Input: part model. Units: mm. Frame: model coordinates. A direction names the side the tool comes from. Coordinates: 2 decimals unless noted, no trailing zeros. Write each loop counter-clockwise with the first axis right and the second up, starting at its lowest first coordinate (ties: lowest second). Pieces come first, ordered by that corner, then holes.
1) Section query A-A (x = 0). Output: boundary loops of the cut face in (y, z).
2) Pin query (flat end, axial travel): pin 1 Ø1.8 at (x, y) = (5.66, -5.66) entering from -Z; pin 2 Ø2 at (x, y) = (7.5, -4.5) entering from +Z. Return the tip coordinate at first contact, or that it passes through.
3) Section query D-D (y = -6.75). State how many separate pieces and enclosed holes the cut face has, then the cut area to 3 significant figures.
4) Set-up query: faces 4 (the flat face through (0, -7, 2)), 5 (the flat face through (0, 3, 0)). Return all of +Z, -Z, +X, -X, +Y, -Y with unobstructed straight access to the full face (end or side cutting, diameter ignored); none if empty.
5) Line query: L1, parallel to Y at x = 0, z = 3; L2, parallel to Z at x = -3.5, y = 6.75; L3, parallel to Y at x = 0.5, z = 3. Output: solid intervals per line, ascending.
6) Section query C-C (z = 4.5). Output: boundary loops of the cut face in (x, y), then the cut area to 3 significant figures.
7) Draft query along X for faces 1 (the flat face through (1, -3, 12)), 2 (the cylindrical face through (-2.38, -10.74, 0.74)), 3 (the cylindrical face through (-4.225, 6.108, 0.986)). Return one class per face: pulls with the +X half, pulls with the -X half, needs draft (parallel to the pull), parting line crosses it, or undercut.
from build123d import *

# Parameters (mm, degrees)
SKETCH1_R           = 11
SKETCH1_R_2         = 2.5
SKETCH1_R_3         = 1.5
BOSS_EXTRUDE1_DEPTH = 2
SKETCH2_R           = 5
SKETCH2_R_2         = 2.5
BOSS_EXTRUDE2_DEPTH = 10
FILLET1_R           = 0.5


with BuildPart() as part:
    # Sketch1 → Boss-Extrude1 (new body)
    with BuildSketch(Plane.XY):
        Circle(SKETCH1_R)
        Circle(SKETCH1_R_2, mode=Mode.SUBTRACT)
        with Locations((-5.655999742, 5.657708628)):
            Circle(SKETCH1_R_3, mode=Mode.SUBTRACT)
        with Locations((5.655999742, 5.657708628)):
            Circle(SKETCH1_R_3, mode=Mode.SUBTRACT)
        with Locations((5.655999742, -5.657708628)):
            Circle(SKETCH1_R_3, mode=Mode.SUBTRACT)
        with Locations((-5.655999742, -5.657708628)):
            Circle(SKETCH1_R_3, mode=Mode.SUBTRACT)
    extrude(amount=BOSS_EXTRUDE1_DEPTH)

    # Sketch2 → Boss-Extrude2 (add)
    with BuildSketch(Plane.XY.offset(2)):
        Circle(SKETCH2_R)
        Circle(SKETCH2_R_2, mode=Mode.SUBTRACT)
    extrude(amount=BOSS_EXTRUDE2_DEPTH)

    # Fillet1
    fillet1_edges = [part.edges().sort_by_distance(p)[0] for p in [
        (-5, 0, 12),
        (-5, 0, 2),
        (-2.5, 0, 12),
        (-11, 0, 2),
    ]]
    fillet(fillet1_edges, radius=FILLET1_R)


solid = part.part
Answer:
1. outline: (-11, 0) - (-2.5, 0) - (-2.5, 11.5) arc R0.5 ccw to (-3, 12) - (-4.5, 12) arc R0.5 ccw to (-5, 11.5) - (-5, 2.5) arc R0.5 cw to (-5.5, 2) - (-10.5, 2) arc R0.5 ccw to (-11, 1.5) - close; (2.5, 0) - (11, 0) - (11, 1.5) arc R0.5 ccw to (10.5, 2) - (5.5, 2) arc R0.5 cw to (5, 2.5) - (5, 11.5) arc R0.5 ccw to (4.5, 12) - (3, 12) arc R0.5 ccw to (2.5, 11.5) - close
2. pin 1: passes through
2. pin 2: stops at z = 2
3. separate pieces: 3
3. enclosed holes: 0
3. area: 26.4 mm2
4. face 4: +Z
4. face 5: -Z, +X, -X, +Y, -Y
5. L1: y = -5 to -2.5, 2.5 to 5
5. L2: z = 0 to 2
5. L3: y = -4.97 to -2.45, 2.45 to 4.97
6. outline: circle Ø10 at (0, 0); hole circle Ø5 at (0, 0)
6. area: 58.9 mm2
7. face 1: needs draft
7. face 2: parting line crosses it
7. face 3: undercut
